Build history of the part. All positions in model axes, mm. Face numbers are marked on the shaded views. A direction names the side the tool comes from. Give positions to 0.01 mm unless a question says otherwise; leave off trailing zeros. Loops run counter-clockwise (first coordinate to the right, second up) from the corner with the lowest first, then second, coordinate; pieces in that order, holes last. Notation, with made-up numbers: (-37.75, 31) -> (8.25, 31) arc R15 ccw to (8.25, 59) -> close; hole circle Ø4 at (21.5, 65). An arc over 180 degrees is marked (long way). Answer as a JSON object with one key per item and string values. Group by question number.
Q1. Drop flat-ended pins along their axis: pin 1 (22 mm diameter, centred on y = -4, z = 10.5, fed in from +X); pin 2 (6 mm diameter, centred on x = -3.5, z = 25, fed in from -Y); pin 3 (19.5 mm diameter, centred on x = 0, y = 0, fed in from -Z); pin 4 (10 mm diameter, centred on x = 52.5, z = -3, fed in from +Y). Give the stop position or say it passes through.
Q2. Band-saw the part on B-B, the plane y = 0. Write the cut outline in (x, z).
Q3. Tool access for the marked faces 5 and 6: list every direction of +Z, -Z, +X, -X, +Y, -Y with a clear straight run to the whole face (end or side of a thin tool).
Q4. Band-saw the part on A-A, the plane z = 30.5. Write the cut outline in (x, y).
Q5. Band-saw the part on D-D, the plane z = 5. Write the cut outline in (x, y), plus the area to 3 significant figures.
Q6. Wall check: probe 1 along X at (y, z) = (0, 22.5); probe 2 along Y at (x, z) = (0, 20.5); probe 3 along Y at (x, z) = (-13, 38.5). Give the ranges that are in metal, low to high. Write a range as from..to.
Q7. Two-plate mould, pull along Z, no slides. Class the marked faces 1, 2, 3 and 4: pulls with the +Z half, pulls with the -Z half, needs draft (parallel to the pull), parting line crosses it, or undercut.
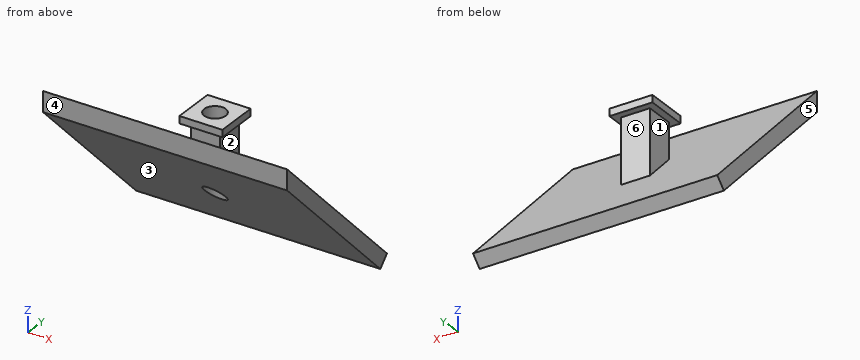
from build123d import *

# Parameters (mm, degrees)
F1_W     = 170
F1_H     = 150
F2_DEPTH = 10
F3_SIZE  = 9.99999
F5_DEPTH = 10
F6_W     = 30
F6_H     = 30
F7_DEPTH = 5
F8_R     = 7.5
F9_DEPTH = 100.1050764009


# Not quite as in the source:
# - a fillet or chamfer is up to 0.001 mm smaller than in the source, because OpenCascade refuses the exact size


with BuildPart() as f2:
    # F1 (on face) → F2 (new body)
    with BuildSketch(Plane(origin=(0, 0, 0), x_dir=(1, 0, 0), z_dir=(0, -0.7071067812, -0.7071067812))):
        Rectangle(F1_W, F1_H)
    extrude(amount=F2_DEPTH)

    # F3 (size 10 in the source; OpenCascade refuses exactly that, so slightly less here)
    f3_edges = [f2.edges().sort_by_distance(p)[0] for p in [
        (0, -60.104076, 45.961941),
    ]]
    chamfer(f3_edges, length=F3_SIZE)

    # F4 (on Right) → F5 (join, symmetric)
    with BuildSketch(Plane.YZ):
        Polygon((-10, 35), (-10, 10), (10, -10), (10, 35), align=None)
    extrude(amount=F5_DEPTH, both=True)

    # F6 (on face) → F7 (join)
    with BuildSketch(Plane.XY.offset(35)):
        Rectangle(F6_W, F6_H)
    extrude(amount=F7_DEPTH)

    # F8 (on face) → F9 (cut, through all)
    with BuildSketch(Plane.XY.offset(40)):
        Circle(F8_R)
    extrude(amount=-F9_DEPTH, mode=Mode.SUBTRACT)


solid = f2.part
Worked answers:
{
 "1": {"pin 1": "x = 85", "pin 2": "y = -42.14", "pin 3": "z = -23.89", "pin 4": "y = 8"},
 "2": {"outline": "(-85, -14.14) -> (-7.5, -14.14) -> (-7.5, 40) -> (-15, 40) -> (-15, 35) -> (-10, 35) -> (-10, 0) -> (-85, 0) -> close; (7.5, -14.14) -> (85, -14.14) -> (85, 0) -> (10, 0) -> (10, 35) -> (15, 35) -> (15, 40) -> (7.5, 40) -> close"},
 "3": {"face 5": "+Z, -Z, -X, +Y, -Y", "face 6": "+X, -X, +Y"},
 "4": {"outline": "(-85, -44.64) -> (85, -44.64) -> (85, -30.5) -> (-85, -30.5) -> close; (-10, -10) -> (10, -10) -> (10, 10) -> (-10, 10) -> close; hole circle Ø15 at (0, 0)"},
 "5": {"outline": "(-85, -19.14) -> (85, -19.14) -> (85, -5) -> (10, -5) -> (10, 10) -> (-10, 10) -> (-10, -5) -> (-85, -5) -> close; hole circle Ø15 at (0, 0)", "area": "2,530 mm2"},
 "6": {"probe 1": "-10..-7.5, 7.5..10", "probe 2": "-34.64..-20.5, -10..-7.5, 7.5..10", "probe 3": "-52.64..-38.5, -15..15"},
 "7": {"face 1": "undercut", "face 2": "undercut", "face 3": "pulls with the -Z half", "face 4": "needs draft"}
}
